For this review, take the finished solid that the model builds, in its own axes (mm). Face numbers are marked on the shaded views. A direction names the side the tool comes from. Give positions to 0.01 mm unless a question says otherwise; leave off trailing zeros. Loops run counter-clockwise (first coordinate to the right, second up) from the corner with the lowest first, then second, coordinate; pieces in that order, holes last.
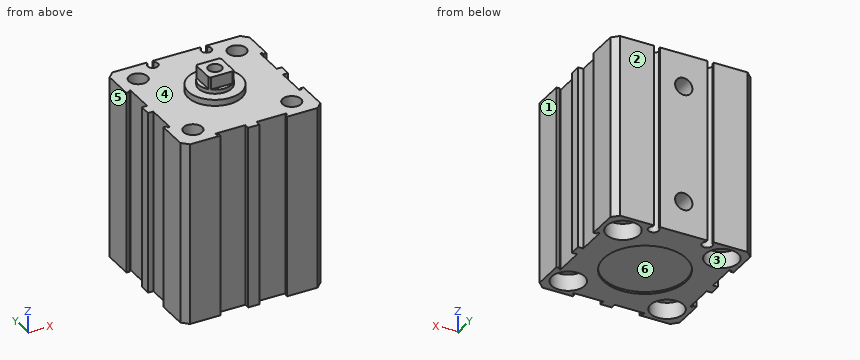
```python
from build123d import *

# Parameters (mm, degrees)
SKETCH_1_W                     = 34
SKETCH_1_H                     = 34
EXTRUDE_1_DEPTH                = 44.5
SKETCH_2_R                     = 10
CUT_EXTRUDE_1_DEPTH            = 0.5
CUT_EXTRUDE_START              = -0.5
SKETCH_3_R                     = 10
CUT_EXTRUDE_2_DEPTH            = 0.5
SKETCH_4_R                     = 4
EXTRUDE_2_DEPTH                = 6
CHAMFER_1_SIZE                 = 1.5
HOLE_WIZARD_M4_1_D             = 4.5
HOLE_WIZARD_M4_1_CBORE_D       = 8
HOLE_WIZARD_M4_1_CBORE_DEPTH   = 4
HOLE_WIZARD_M4_1_2_D           = 3.3
HOLE_WIZARD_M4_1_2_DEPTH       = 10.1
HOLE_WIZARD_M4_1_2_TIP         = 0.991420021
SKETCH_9_W                     = 5.05425195
SKETCH_9_H                     = 13.3836291
SKETCH_9_W_2                   = 3.579653673
SKETCH_9_H_2                   = 11.317985889
CUT_EXTRUDE_3_DEPTH            = 3
SKETCH_14_R                    = 1.25
CUT_EXTRUDE_6_DEPTH            = 51.5791459
SKETCH_15_W                    = 1.5
SKETCH_15_H                    = 1
CUT_EXTRUDE_7_DEPTH            = 51.5791459
PATTERN_CIRCULAR_1_COUNT       = 2
PATTERN_CIRCULAR_1_ANGLE       = 90
SKETCH_16_R                    = 6.5
SKETCH_16_R_2                  = 1.65
EXTRUDE_3_DEPTH                = 2
EXTRUDE_START                  = 0.5
SKETCH_17_R                    = 10
SKETCH_17_R_2                  = 1.65
EXTRUDE_4_DEPTH                = 0.5
SKETCH_18_W                    = 1.251760675
SKETCH_18_H                    = 6.736418335
CUT_EXTRUDE_8_DEPTH            = 51.5791459
SKETCH_19_W                    = 0.490453646
SKETCH_19_H                    = 0.506695446
CUT_EXTRUDE_9_DEPTH            = 51.5791459
PATTERN_START                  = -17
PATTERN_CIRCULAR_2_OUTLINE_W   = 6.736418335
PATTERN_CIRCULAR_2_OUTLINE_H   = 44.5
PATTERN_CIRCULAR_2_DEPTH       = 1.251760675
PATTERN_START_2                = -8.103506379
PATTERN_CIRCULAR_2_2_OUTLINE_W = 1.251760675
PATTERN_CIRCULAR_2_2_OUTLINE_H = 44.5
PATTERN_CIRCULAR_2_2_DEPTH     = 6.736418335
PATTERN_START_3                = 1.367088044
PATTERN_CIRCULAR_2_3_OUTLINE_W = 1.251760675
PATTERN_CIRCULAR_2_3_OUTLINE_H = 44.5
PATTERN_CIRCULAR_2_3_DEPTH     = 6.736418335
PATTERN_START_4                = -16.238692971
PATTERN_CIRCULAR_2_4_OUTLINE_W = 0.506695446
PATTERN_CIRCULAR_2_4_OUTLINE_H = 44.5
PATTERN_CIRCULAR_2_4_DEPTH     = 0.490453646
PATTERN_START_5                = -8.610201825
PATTERN_CIRCULAR_2_5_OUTLINE_W = 0.490453646
PATTERN_CIRCULAR_2_5_OUTLINE_H = 44.5
PATTERN_CIRCULAR_2_5_DEPTH     = 0.506695446
PATTERN_START_6                = 8.103506379
PATTERN_CIRCULAR_2_6_OUTLINE_W = 0.490453646
PATTERN_CIRCULAR_2_6_OUTLINE_H = 44.5
PATTERN_CIRCULAR_2_6_DEPTH     = 0.506695446
HOLE_WIZARD_M5_1_D             = 4.2
HOLE_WIZARD_M5_1_DEPTH         = 12.4
HOLE_WIZARD_M5_1_TIP           = 1.2618073


# Read off the part's stored shape, not the designer's step: 阵列(圆周)2
with BuildPart() as part:
    # 草图1 → 凸台-拉伸1 (new body)
    with BuildSketch(Plane.XY):
        Rectangle(SKETCH_1_W, SKETCH_1_H)
    extrude(amount=EXTRUDE_1_DEPTH)

    # 草图2 → 切除-拉伸1 (cut)
    with BuildSketch(Plane.XY.offset(44.5)):
        Circle(SKETCH_2_R)
    extrude(amount=-CUT_EXTRUDE_1_DEPTH, mode=Mode.SUBTRACT)

    # 草图3 → 切除-拉伸2 (cut)
    with BuildSketch(Plane(origin=(0, 0, 0), x_dir=(-1, 0, 0), z_dir=(0, 0, -1)).offset(CUT_EXTRUDE_START)):
        with Locations(Location((0, 0, 0), (0, 0, 180))):
            Circle(SKETCH_3_R)
    extrude(amount=CUT_EXTRUDE_2_DEPTH, mode=Mode.SUBTRACT)

    # 草图4 → 凸台-拉伸2 (add)
    with BuildSketch(Plane.XY.offset(44)):
        Circle(SKETCH_4_R)
    extrude(amount=EXTRUDE_2_DEPTH)

    # 倒角1
    chamfer_1_edges = [part.edges().sort_by_distance(p)[0] for p in [
        (-17, 17, 22.25),
        (17, 17, 22.25),
        (17, -17, 22.25),
        (-17, -17, 22.25),
    ]]
    chamfer(chamfer_1_edges, length=CHAMFER_1_SIZE)

    # Hole Wizard M4 _1 (through all)
    with Locations(Plane(origin=(0, 0, 0), x_dir=(-1, 0, 0), z_dir=(0, 0, -1))):
        with Locations((-12, 12), (12, -12), (12, 12), (-12, -12)):
            CounterBoreHole(HOLE_WIZARD_M4_1_D / 2, HOLE_WIZARD_M4_1_CBORE_D / 2, HOLE_WIZARD_M4_1_CBORE_DEPTH)

    # Hole Wizard M4 _1 2
    with Locations(Plane.XY.offset(50)):
        with Locations((0, 0)):
            Hole(HOLE_WIZARD_M4_1_2_D / 2, depth=HOLE_WIZARD_M4_1_2_DEPTH)
            with Locations((0, 0, -(HOLE_WIZARD_M4_1_2_DEPTH + HOLE_WIZARD_M4_1_2_TIP / 2))):  # 118° drill point
                Cone(0, HOLE_WIZARD_M4_1_2_D / 2, HOLE_WIZARD_M4_1_2_TIP, mode=Mode.SUBTRACT)

    # 草图9 → 切除-拉伸3 (cut)
    with BuildSketch(Plane.XY.offset(50)):
        with Locations((-5.527125975, -0.54919334)):
            Rectangle(SKETCH_9_W, SKETCH_9_H)
        with Locations((4.789826836, -0.152935728)):
            Rectangle(SKETCH_9_W_2, SKETCH_9_H_2)
    cut_extrude_3 = extrude(amount=-CUT_EXTRUDE_3_DEPTH, mode=Mode.SUBTRACT)

    # 草图14 → 切除-拉伸6 (cut, through all)
    with BuildSketch(Plane.XY.offset(44.5)):
        with Locations((-6.5, 15.5)):
            Circle(SKETCH_14_R)
        with Locations(Location((6.5, 15.5, 0), (0, 0, 180))):
            Circle(SKETCH_14_R)
    extrude(amount=-CUT_EXTRUDE_6_DEPTH, mode=Mode.SUBTRACT)

    # 草图15 → 切除-拉伸7 (cut, through all)
    with BuildSketch(Plane.XY.offset(44.5)):
        with Locations((-6.5, 16.5)):
            Rectangle(SKETCH_15_W, SKETCH_15_H)
        with Locations((6.5, 16.5)):
            Rectangle(SKETCH_15_W, SKETCH_15_H)
    extrude(amount=-CUT_EXTRUDE_7_DEPTH, mode=Mode.SUBTRACT)

    # 阵列(圆周)1: 切除-拉伸3 ×2 about axis
    pattern_circular_1_axis = Axis((0, 0, 50), (0, 0, -1))
    for i in range(1, PATTERN_CIRCULAR_1_COUNT):
        add(cut_extrude_3.rotate(pattern_circular_1_axis, i * PATTERN_CIRCULAR_1_ANGLE / (PATTERN_CIRCULAR_1_COUNT - 1)), mode=Mode.SUBTRACT)

    # 草图16 → 凸台-拉伸3 (add)
    with BuildSketch(Plane.XY.offset(44)):
        Circle(SKETCH_16_R)
        Circle(SKETCH_16_R_2, mode=Mode.SUBTRACT)
    extrude(amount=EXTRUDE_3_DEPTH)

    # 草图17 → 凸台-拉伸4 (add)
    with BuildSketch(Plane.XY.offset(44).offset(EXTRUDE_START)):
        with Locations(Location((0, 0, 0), (0, 0, 180))):
            Circle(SKETCH_17_R)
        Circle(SKETCH_17_R_2, mode=Mode.SUBTRACT)
    extrude(amount=-EXTRUDE_4_DEPTH)

    # 草图18 → 切除-拉伸8 (cut, through all)
    with BuildSketch(Plane.XY.offset(44.5)):
        with Locations((16.374119663, 4.735297212)):
            Rectangle(SKETCH_18_W, SKETCH_18_H)
        with Locations((16.374119663, -4.735297212)):
            Rectangle(SKETCH_18_W, SKETCH_18_H)
    extrude(amount=-CUT_EXTRUDE_8_DEPTH, mode=Mode.SUBTRACT)

    # 草图19 → 切除-拉伸9 (cut, through all)
    with BuildSketch(Plane.XY.offset(44.5)):
        with Locations((15.993466148, 8.356854102)):
            Rectangle(SKETCH_19_W, SKETCH_19_H)
        with Locations((15.993466148, -8.356854102)):
            Rectangle(SKETCH_19_W, SKETCH_19_H)
    extrude(amount=-CUT_EXTRUDE_9_DEPTH, mode=Mode.SUBTRACT)

    # 阵列(圆周)2 outline → 阵列(圆周)2 (cut)
    with BuildSketch(Plane(origin=(0, 0, 0), x_dir=(1, 0, 0), z_dir=(0, 1, 0)).offset(PATTERN_START)):
        with Locations((4.735297212, -22.25)):
            Rectangle(PATTERN_CIRCULAR_2_OUTLINE_W, PATTERN_CIRCULAR_2_OUTLINE_H)
        with Locations((-4.735297212, -22.25)):
            Rectangle(PATTERN_CIRCULAR_2_OUTLINE_W, PATTERN_CIRCULAR_2_OUTLINE_H)
    extrude(amount=PATTERN_CIRCULAR_2_DEPTH, mode=Mode.SUBTRACT)

    # Pattern Circular 2 2 outline → Pattern Circular 2 2 (cut)
    with BuildSketch(Plane(origin=(0, 0, 0), x_dir=(1, 0, 0), z_dir=(0, 1, 0)).offset(PATTERN_START_2)):
        with Locations((-16.374119663, -22.25)):
            Rectangle(PATTERN_CIRCULAR_2_2_OUTLINE_W, PATTERN_CIRCULAR_2_2_OUTLINE_H)
    extrude(amount=PATTERN_CIRCULAR_2_2_DEPTH, mode=Mode.SUBTRACT)

    # Pattern Circular 2 3 outline → Pattern Circular 2 3 (cut)
    with BuildSketch(Plane(origin=(0, 0, 0), x_dir=(1, 0, 0), z_dir=(0, 1, 0)).offset(PATTERN_START_3)):
        with Locations((-16.374119663, -22.25)):
            Rectangle(PATTERN_CIRCULAR_2_3_OUTLINE_W, PATTERN_CIRCULAR_2_3_OUTLINE_H)
    extrude(amount=PATTERN_CIRCULAR_2_3_DEPTH, mode=Mode.SUBTRACT)

    # Pattern Circular 2 4 outline → Pattern Circular 2 4 (cut)
    with BuildSketch(Plane(origin=(0, 0, 0), x_dir=(1, 0, 0), z_dir=(0, 1, 0)).offset(PATTERN_START_4)):
        with Locations((8.356854102, -22.25)):
            Rectangle(PATTERN_CIRCULAR_2_4_OUTLINE_W, PATTERN_CIRCULAR_2_4_OUTLINE_H)
        with Locations((-8.356854102, -22.25)):
            Rectangle(PATTERN_CIRCULAR_2_4_OUTLINE_W, PATTERN_CIRCULAR_2_4_OUTLINE_H)
    extrude(amount=PATTERN_CIRCULAR_2_4_DEPTH, mode=Mode.SUBTRACT)

    # Pattern Circular 2 5 outline → Pattern Circular 2 5 (cut)
    with BuildSketch(Plane(origin=(0, 0, 0), x_dir=(1, 0, 0), z_dir=(0, 1, 0)).offset(PATTERN_START_5)):
        with Locations((-15.993466148, -22.25)):
            Rectangle(PATTERN_CIRCULAR_2_5_OUTLINE_W, PATTERN_CIRCULAR_2_5_OUTLINE_H)
    extrude(amount=PATTERN_CIRCULAR_2_5_DEPTH, mode=Mode.SUBTRACT)

    # Pattern Circular 2 6 outline → Pattern Circular 2 6 (cut)
    with BuildSketch(Plane(origin=(0, 0, 0), x_dir=(1, 0, 0), z_dir=(0, 1, 0)).offset(PATTERN_START_6)):
        with Locations((-15.993466148, -22.25)):
            Rectangle(PATTERN_CIRCULAR_2_6_OUTLINE_W, PATTERN_CIRCULAR_2_6_OUTLINE_H)
    extrude(amount=PATTERN_CIRCULAR_2_6_DEPTH, mode=Mode.SUBTRACT)

    # M5 螺纹孔1
    with Locations(Plane(origin=(0, 17, 0), x_dir=(-1, 0, 0), z_dir=(0, 1, 0))):
        with Locations((0, 36.5), (0, 8)):
            Hole(HOLE_WIZARD_M5_1_D / 2, depth=HOLE_WIZARD_M5_1_DEPTH)
            with Locations((0, 0, -(HOLE_WIZARD_M5_1_DEPTH + HOLE_WIZARD_M5_1_TIP / 2))):  # 118° drill point
                Cone(0, HOLE_WIZARD_M5_1_D / 2, HOLE_WIZARD_M5_1_TIP, mode=Mode.SUBTRACT)


solid = part.part
```
Q1. Mouldability with a two-part tool opening along Y and no side actions: class the marked faces 1, 2 and 3 as +Y half, -Y half, draft (parallel to the pull), parting line (faces both ways), or undercut.
Answers:
face 1: draft
face 2: +Y half
face 3: undercut
Q2. Machinability: for the marked faces 4, 5 and 6, which of the approach directions +Z, -Z, +X, -X, +Y, -Y give a long, thin tool a straight path to every point of the face, cutting with its end or side? Answer none if there is none.
Answers:
face 4: +Z
face 5: +Z, -Z, -X, +Y, -Y
face 6: -Z
Q3. For probe 1 along Y at (x, z) = (-12, 13.5); probe 2 along X at (y, z) = (8.5, 33.5); probe 3 along X at (y, z) = (-14, 26.5), list the stretches that pass through material, from the lowest coordinate up.
Answers:
probe 1: y = -17 to -14.25, -9.75 to 9.75, 14.25 to 17
probe 2: x = -17 to -16.24, -15.75 to 15.75, 16.24 to 17
probe 3: x = -17 to -13.03, -10.97 to 10.97, 13.03 to 17
Q4. Consider section C-C on y = 5.5. Give the boundary of the cut face in (x, z).
Answers:
outline: (-15.75, 0) - (-8.35, 0) - (-8.35, 0.5) - (8.35, 0.5) - (8.35, 0) - (15.75, 0) - (15.75, 44.5) - (3.46, 44.5) - (3.46, 46) - (-3.46, 46) - (-3.46, 44.5) - (-15.75, 44.5) - close; hole circle Ø4.2 at (0, 8); hole circle Ø4.2 at (0, 36.5)
Q5. Consider section B-B on y = 13. Give the boundary of the cut face in (x, z), plus the area to 3 significant figures.
Answers:
outline: (-17, 0) - (-15.87, 0) - (-15.87, 4) - (-14.02, 4) - (-14.02, 44.5) - (-17, 44.5) - close; (-9.98, 4) - (-8.13, 4) - (-8.13, 0) - (8.13, 0) - (8.13, 4) - (9.98, 4) - (9.98, 44.5) - (-9.98, 44.5) - close; (14.02, 4) - (15.87, 4) - (15.87, 0) - (17, 0) - (17, 44.5) - (14.02, 44.5) - close; hole circle Ø4.2 at (0, 8); hole circle Ø4.2 at (0, 36.5)
area: 1,100 mm2
Q6. Consider section D-D on z = 42.5. Count the separate pieces of the cut face and the enclosed holes in it, plus the area to 3 significant figures.
Answers:
separate pieces: 1
enclosed holes: 5
area: 1,020 mm2
Q7. For pin 1 Ø5 at (x, y) = (12, 12) entering from -Z; pin 2 Ø8 at (x, y) = (11, -3) entering from +Z; pin 3 Ø1 at (x, z) = (3, 32) entering from -Y, all flat-tipped, find the tip position at first contact; note any pin that passes through.
Answers:
pin 1: stops at z = 4
pin 2: stops at z = 44.5
pin 3: stops at y = -15.75
Q8. Consider section A-A on x = -12. Give the boundary of the cut face in (y, z).
Answers:
outline: (-17, 0) - (-16, 0) - (-16, 4) - (-14.25, 4) - (-14.25, 44.5) - (-17, 44.5) - close; (-9.75, 4) - (-8, 4) - (-8, 0) - (8, 0) - (8, 4) - (9.75, 4) - (9.75, 44.5) - (-9.75, 44.5) - close; (14.25, 4) - (16, 4) - (16, 0) - (17, 0) - (17, 44.5) - (14.25, 44.5) - close
